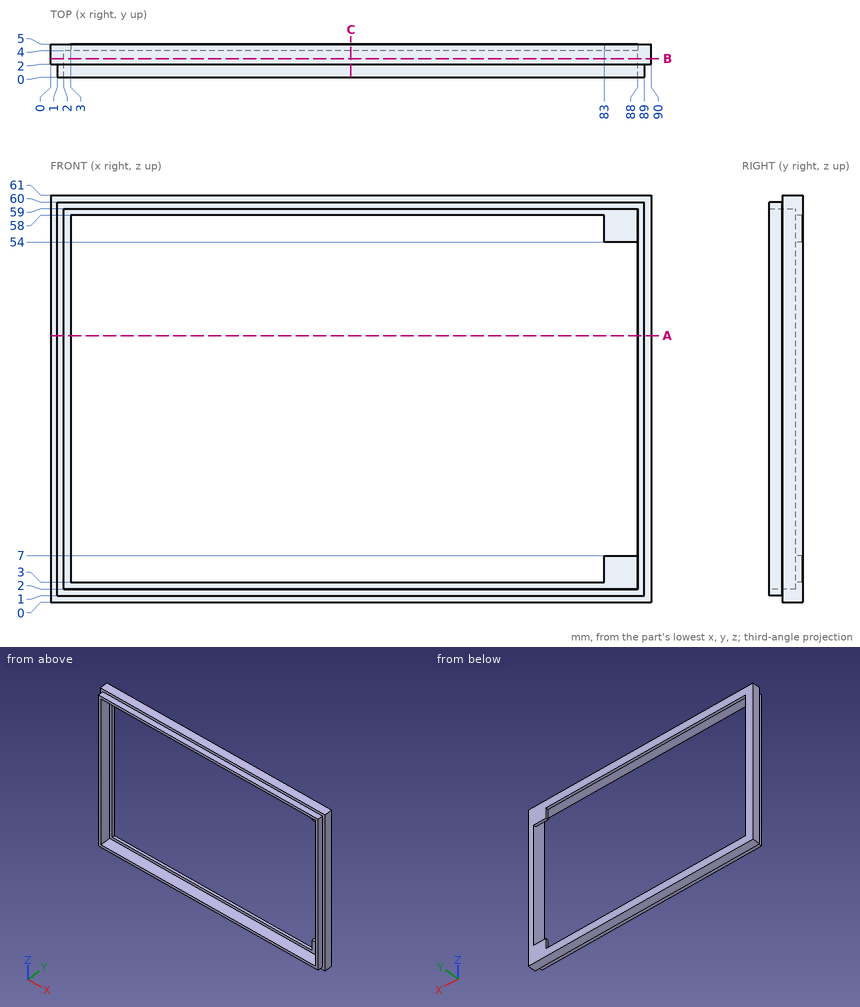
Geometry check sheet. Reference: drawing and pictorial views, mm from the part's lowest x, y, z. Give positions to 0.01 mm unless a question says otherwise; leave off trailing zeros. Order: outer loops, then holes, each group sorted by start corner. A loop starts at its lowest first (then second) coordinate and runs counter-clockwise, first axis right, second up. Notation, with made-up numbers: M -1.5,37 L 48.5,37 A31 cw 48.5,75 Z; hole C -27,30 d8. An arc over 180 degrees is marked long. Answer as a JSON object with one key per item and string values. Group by question number.
1) Cross-section at B-B (y = 2.8). Enter the section's corners in (x, z).
2) Scan lines: line 1 along X through (y, z) = (1.25, 33); line 2 along Z through (x, y) = (21, 1.8); line 3 along Z through (x, y) = (43.5, 4.8). Record each from-to range of solid material in increasing order. Write a range as [from, to].
3) Cross-section at A-A (z = 40). Enter the section's corners in (x, y).
4) Cross-section at C-C (x = 45). Enter the section's corners in (y, z), then the cut area to 3 significant figures.
5) Depth check by flat-ended pin: pin 1 Ø1.2 at (x, y) = (26, 2) entering from -Z; pin 2 Ø1.6 at (x, y) = (51.5, 1) entering from +Z; pin 3 Ø2 at (y, z) = (0.5, 25.5) entering from +X; pin 4 Ø2 at (x, y) = (30.5, 0.5) entering from -Z. Enter the tip coordinate at first touch or a pass-through.
Result sheet:
{
 "1": {"outline": "M 0,0 L 90,0 L 90,61 L 0,61 Z; hole M 2,2 L 88,2 L 88,59 L 2,59 Z"},
 "2": {"line 1": "x = [1, 2], [88, 89]", "line 2": "z = [1, 2], [59, 60]", "line 3": "z = [0, 3], [58, 61]"},
 "3": {"outline": "M 0,2 L 1,2 L 1,0 L 2,0 L 2,4 L 3,4 L 3,5 L 0,5 Z; M 88,0 L 89,0 L 89,2 L 90,2 L 90,5 L 88,5 Z"},
 "4": {"outline": "M 0,1 L 2,1 L 2,0 L 5,0 L 5,3 L 4,3 L 4,2 L 0,2 Z; M 0,59 L 4,59 L 4,58 L 5,58 L 5,61 L 2,61 L 2,60 L 0,60 Z", "area": "18.0 mm2"},
 "5": {"pin 1": "stops at z = 0", "pin 2": "stops at z = 60", "pin 3": "stops at x = 89", "pin 4": "stops at z = 1"}
}
